Can you work these out from the model? Positions are in its coordinate system, mm. Face numbers are marked on the shaded views. Coordinates: 2 decimals unless noted, no trailing zeros. Loops run counter-clockwise (first coordinate to the right, second up) from the corner with the lowest first, then second, coordinate; pieces in that order, holes last.
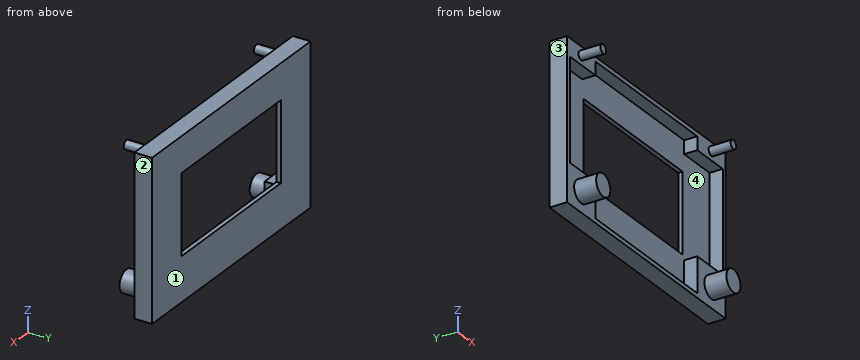
```python
from build123d import *

# Parameters (mm, degrees)
SKETCH_1_W      = 56
SKETCH_1_H      = 36
EXTRUDE_3_DEPTH = 3
SKETCH_2_W      = 56
SKETCH_2_H      = 36
SKETCH_2_W_2    = 35
SKETCH_2_H_2    = 18
EXTRUDE_4_DEPTH = 1
SKETCH_3_R      = 1
SKETCH_3_R_2    = 2.5
EXTRUDE_5_DEPTH = 5


with BuildPart() as part:
    # 草图1 → 凸台-拉伸3 (new body)
    with BuildSketch(Plane(origin=(0, 0, 0), x_dir=(1, 0, 0), z_dir=(0, 1, 0))):
        with Locations((28, -18)):
            Rectangle(SKETCH_1_W, SKETCH_1_H)
        Polygon((10, -32), (1, -32), (1, -9), (10, -9), (10, -1), (46, -1), (46, -9), (55, -9), (55, -32), (46, -32), (46, -35), (10, -35), align=None, mode=Mode.SUBTRACT)
    extrude(amount=EXTRUDE_3_DEPTH)

    # 草图2 → 凸台-拉伸4 (add)
    with BuildSketch(Plane(origin=(0, 3, 0), x_dir=(1, 0, 0), z_dir=(0, 1, 0))):
        with Locations((28, -18)):
            Rectangle(SKETCH_2_W, SKETCH_2_H)
        with Locations((28, -19)):
            Rectangle(SKETCH_2_W_2, SKETCH_2_H_2, mode=Mode.SUBTRACT)
    extrude(amount=EXTRUDE_4_DEPTH)

    # 草图3 → 凸台-拉伸5 (add)
    with BuildSketch(Plane(origin=(0, 0, 0), x_dir=(-1, 0, 0), z_dir=(0, -1, 0))):
        with Locations(Location((-51, -34, 0), (0, 0, 270))):
            Circle(SKETCH_3_R)
        with Locations(Location((-5, -34, 0), (0, 0, 270))):
            Circle(SKETCH_3_R)
        with Locations(Location((-51, -4.5, 0), (0, 0, 270))):
            Circle(SKETCH_3_R_2)
        with Locations(Location((-5, -4.5, 0), (0, 0, 270))):
            Circle(SKETCH_3_R_2)
    extrude(amount=EXTRUDE_5_DEPTH)


solid = part.part
```
(1) I want a section at B-B on x = 33. Write out the boundary of the cut face in (y, z).
Check values:
outline: (0, 0) - (4, 0) - (4, 10) - (3, 10) - (3, 1) - (0, 1) - close; (0, 35) - (3, 35) - (3, 28) - (4, 28) - (4, 36) - (0, 36) - close
(2) I want a section at A-A on z = 23.5. Write out the boundary of the cut face in (x, y).
Check values:
outline: (0, 0) - (1, 0) - (1, 3) - (10.5, 3) - (10.5, 4) - (0, 4) - close; (45.5, 3) - (55, 3) - (55, 0) - (56, 0) - (56, 4) - (45.5, 4) - close
(3) If I drill on probe 1 along Z at (x, y) = (51, -4.25); probe 2 along Z at (x, y) = (23.5, 0.5); probe 3 along X at (y, z) = (0.25, 24.5), over which ranges is the centre line in solid material (lowest first)?
Check values:
probe 1: z = 2 to 7, 33 to 35
probe 2: z = 0 to 1, 35 to 36
probe 3: x = 0 to 1, 55 to 56
(4) If we mould it in two halves opening along X, with no side actions, what happens to the marked faces 1, 2, 3 and 4? For each: released by +X, released by -X, zero draft, split by the parting line, or undercut.
Check values:
face 1: zero draft
face 2: released by +X
face 3: released by -X
face 4: undercut
(5) I'm going to push a flat-ended pin straight in: pin 1 (2 mm diameter, centred on y = -2.5, z = 31.5, fed in from -X). Where does the tip first touch, or does it pass through?
Check values:
pin 1: passes through
(6) I want a section at D-D on z = 34. Write out the boundary of the cut face in (x, y).
Check values:
outline: (0, 0) - (4, 0) - (4, -5) - (6, -5) - (6, 0) - (10, 0) - (10, 3) - (46, 3) - (46, 0) - (50, 0) - (50, -5) - (52, -5) - (52, 0) - (56, 0) - (56, 4) - (0, 4) - close
(7) I want a section at C-C on x = 51. Write out the boundary of the cut face in (y, z), then the cut area to 3 significant figures.
Check values:
outline: (-5, 2) - (0, 2) - (0, 0) - (4, 0) - (4, 36) - (0, 36) - (0, 35) - (-5, 35) - (-5, 33) - (0, 33) - (0, 32) - (3, 32) - (3, 9) - (0, 9) - (0, 7) - (-5, 7) - close
area: 110 mm2
